```python
from build123d import *

# Parameters (mm, degrees)
BOSS_EXTRUDE1_DEPTH = 19.999999553
CUT_EXTRUDE1_DEPTH  = 158.443784597
CUT_EXTRUDE2_DEPTH  = 158.443784597
SKETCH7_W           = 15.825305434
SKETCH7_H           = 12.213007454
SKETCH7_W_2         = 10.489088449
SKETCH7_H_2         = 8.460664219
BOSS_EXTRUDE5_DEPTH = 20
SKETCH6_R           = 3.982936417
SKETCH6_R_2         = 3.990480896
CUT_EXTRUDE8_DEPTH  = 40
SKETCH8_W           = 26.734403149
SKETCH8_H           = 11.210794898
CUT_EXTRUDE9_DEPTH  = 30
FILLET1_R           = 5
FILLET2_R           = 5
SKETCH9_W           = 67.375066669
SKETCH9_H           = 11.734562751
CUT_EXTRUDE10_DEPTH = 8


with BuildPart() as part:
    # Sketch1 → Boss-Extrude1 (new body)
    with BuildSketch(Plane(origin=(0, 0, 0), x_dir=(-1, 0, 0), z_dir=(0, 0, -1))):
        Polygon((150.224894285, 11.525735259), (149.094194174, 12.437307276), (147.882685065, 13.238362968), (146.601140499, 13.921783306), (145.260930061, 14.481496066), (143.87395978, 14.912526123), (-3.873967333, 14.912526123), (-5.275767762, 14.476095326), (-6.629663985, 13.908221386), (-7.923361845, 13.214060105), (-9.145116434, 12.399914674), (-10.28383337, 11.473178864), (-11.329172179, 10.442265309), (-12.271642685, 9.316536598), (-13.102686033, 8.106213063), (-13.814756647, 6.822284777), (-14.401388355, 5.476410501), (-14.857255854, 4.080810118), (-15.178218484, 2.648155671), (-15.361363068, 1.191455987), (-15.405026264, -0.276062055), (-15.308812261, -1.741073444), (-15.073592775, -3.19027598), (-14.70150426, -4.610510543), (-14.195927419, -5.988881458), (-13.561449945, -7.312873378), (-12.803834863, -8.570464328), (-11.929960921, -9.750235826), (-10.947762057, -10.841473937), (129.052236676, -10.841473937), (130.121722817, -11.824152432), (131.278976798, -12.701761909), (132.513716817, -13.466504402), (133.815005422, -14.111584984), (135.171234608, -14.631270431), (136.570379138, -15.020942315), (137.999981642, -15.277140774), (139.447391033, -15.39758686), (140.899673104, -15.381210484), (142.343983054, -15.228157863), (143.767461181, -14.939788729), (145.157456398, -14.518666081), (146.501630545, -13.968531042), (147.788017988, -13.294272125), (149.00521934, -12.501881458), (150.142401457, -11.59839984), (151.189431548, -10.591856204), (152.137070894, -9.49119404), (152.976840734, -8.306192234), (153.701290488, -7.047383115), (154.303997755, -5.725951865), (154.779613018, -4.353639204), (155.123889446, -2.9426408), (155.333772302, -1.505494351), (155.407398939, -0.054970031), (155.344113708, 1.39604276), (155.144497752, 2.834650222), (154.81030941, 4.248069134), (154.344499111, 5.623740144), (153.751239181, 6.949439179), (153.035759926, 8.21338594), (152.204483747, 9.40434821), (151.264742017, 10.511744767), align=None)
    extrude(amount=-BOSS_EXTRUDE1_DEPTH)

    # Sketch2 → Cut-Extrude1 (cut, through all)
    with BuildSketch(Plane.XY.offset(19.999999553)):
        Polygon((3.729888937, 1.444966649), (3.400868736, 2.105728723), (2.956035547, 2.694782568), (2.410538495, 3.192068776), (1.78295339, 3.580653109), (1.094651991, 3.847302636), (0.369073445, 3.982936498), (-0.369073445, 3.982936498), (-1.094651991, 3.847302636), (-1.78295339, 3.580653109), (-2.410538495, 3.192068776), (-2.956035547, 2.694782568), (-3.400868736, 2.105728723), (-3.729888937, 1.444966649), (-3.93189257, 0.73499803), (-4.00000019, 0), (-3.93189257, -0.73499803), (-3.729888937, -1.444966649), (-3.400868736, -2.105728723), (-2.956035547, -2.694782568), (-2.410538495, -3.192068776), (-1.78295339, -3.580653109), (-1.094651991, -3.847302636), (-0.369073445, -3.982936498), (0.369073445, -3.982936498), (1.094651991, -3.847302636), (1.78295339, -3.580653109), (2.410538495, -3.192068776), (2.956035547, -2.694782568), (3.400868736, -2.105728723), (3.729888937, -1.444966649), (3.93189257, -0.73499803), (4.00000019, 0), (3.93189257, 0.73499803), align=None)
    extrude(amount=-CUT_EXTRUDE1_DEPTH, mode=Mode.SUBTRACT)

    # Sketch3 → Cut-Extrude2 (cut, through all)
    with BuildSketch(Plane.XY.offset(19.999999553)):
        Polygon((-139.630913734, 3.982936498), (-140.369072556, 3.982936498), (-141.094654799, 3.847302636), (-141.782954335, 3.580653109), (-142.41053164, 3.192068776), (-142.956033349, 2.694782568), (-143.400862813, 2.105728723), (-143.729895353, 1.444966649), (-143.931895494, 0.73499803), (-143.999993801, 0), (-143.931895494, -0.73499803), (-143.729895353, -1.444966649), (-143.400862813, -2.105728723), (-142.956033349, -2.694782568), (-142.41053164, -3.192068776), (-141.782954335, -3.580653109), (-141.094654799, -3.847302636), (-140.369072556, -3.982936498), (-139.630913734, -3.982936498), (-138.905346394, -3.847302636), (-138.217046857, -3.580653109), (-137.589469552, -3.192068776), (-137.043967843, -2.694782568), (-136.599138379, -2.105728723), (-136.270105839, -1.444966649), (-136.068105698, -0.73499803), (-136.000007391, 0), (-136.068105698, 0.73499803), (-136.270105839, 1.444966649), (-136.599138379, 2.105728723), (-137.043967843, 2.694782568), (-137.589469552, 3.192068776), (-138.217046857, 3.580653109), (-138.905346394, 3.847302636), align=None)
    extrude(amount=-CUT_EXTRUDE2_DEPTH, mode=Mode.SUBTRACT)

    # Sketch7 → Boss-Extrude5 (add)
    with BuildSketch(Plane.XY.offset(19.999999553)):
        with Locations((-139.666933083, -0.328537463)):
            Rectangle(SKETCH7_W, SKETCH7_H)
        with Locations((0.16180396, 0.00184402)):
            Rectangle(SKETCH7_W_2, SKETCH7_H_2)
    extrude(amount=-BOSS_EXTRUDE5_DEPTH)

    # Sketch6 → Cut-Extrude8 (cut)
    with BuildSketch(Plane(origin=(0, 0, -10), x_dir=(-1, 0, 0), z_dir=(0, 0, -1))):
        with Locations((4.82e-07, 8.1e-08)):
            Circle(SKETCH6_R)
        with Locations((140.006757016, -0.008937853)):
            Circle(SKETCH6_R_2)
    extrude(amount=-CUT_EXTRUDE8_DEPTH, mode=Mode.SUBTRACT)

    # Sketch8 → Cut-Extrude9 (cut)
    with BuildSketch(Plane.XY.offset(19.999999553)):
        with Locations((-96.813347326, 9.307128674)):
            Rectangle(SKETCH8_W, SKETCH8_H)
    extrude(amount=-CUT_EXTRUDE9_DEPTH, mode=Mode.SUBTRACT)

    # Fillet1
    fillet1_edges = [part.edges().sort_by_distance(p)[0] for p in [
        (-83.446145751, 3.701731225, 9.999999776),
        (-110.1805489, 3.701731225, 9.999999776),
    ]]
    fillet(fillet1_edges, radius=FILLET1_R)

    # Fillet2
    fillet2_edges = [part.edges().sort_by_distance(p)[0] for p in [
        (-83.446145751, 14.912526123, 9.999999776),
        (-110.1805489, 14.912526123, 9.999999776),
    ]]
    fillet(fillet2_edges, radius=FILLET2_R)

    # Sketch9 → Cut-Extrude10 (cut)
    with BuildSketch(Plane(origin=(0, 2.549240283, 0), x_dir=(-1, 0, 0), z_dir=(0, 0, -1))):
        with Locations((40.062197326, -0.800943257)):
            Rectangle(SKETCH9_W, SKETCH9_H)
    extrude(amount=-CUT_EXTRUDE10_DEPTH, mode=Mode.SUBTRACT)


solid = part.part
```
Could you check a few things on this model? Use its own coordinates, in mm. A direction names the side the tool comes from. Round coordinates to 2 decimals unless told otherwise and drop trailing zeros. Order: outer loops, then holes, each group sorted by start corner. A loop starts at its lowest first (then second) coordinate and runs counter-clockwise, first axis right, second up. Notation, with made-up numbers: M -25.75,-14.75 L 2.25,-14.75 A23 cw 2.25,-6.75 Z; hole C 34,18.5 d1. An arc over 180 degrees is marked long. One line per question, with ' | ' between items. Start each with the question number.
(1) Suppose I cut it at C-C on z = 16. Count the separate pieces of the cut face and the enclosed holes in it, then the cut area to 3 significant figures.
(2) Suppose I cut it at A-A on x = 0. List the corners of the cut face in (y, z) for me.
(3) For faces 1 (the face through (-136.02, 0.17, 9.86)), 2 (the face through (-40, 2, 8)), 3 (the face through (-58, -10.841, 10)), 4 (the face through (-97, 3.702, 10)), which set-ups out of +Z, -Z, +X, -X, +Y, -Y let a thin tool reach every point of the face, with its end or its side?
(4) Thinking about a two-plate mould opening in Y: for faces 5 (the face through (-69, 0, 20)), 6 (the face through (0.86, -3.89, 9.86)), 7 (the face through (-130, 14.913, 10)), which applies, +Y half, -Y half, draft (parallel to the pull), parting line (faces both ways), or undercut?
(5) For P1, Ø9, axis at x = -56.5, z = 5, coming from the -Y side; P2, Ø4, axis at y = -10, z = 16, coming from the -X side; P3, Ø6, axis at y = 8, z = 6.5, coming from the +X side; P4, Ø7, axis at x = -140.01, y = -0.01, coming from the +Z side, each with a flat end and sliding along its axis, tell me the tip position at first contact or that it passes through.
(6) Suppose I cut it at B-B on x = -51. List the corners of the cut face in (y, z) for me, then the cut area to 3 significant figures.
(7) Please list where these lines run through material, in increasing order: line 1 along Y through (x, z) = (-19.5, 3.25); line 2 along Y through (x, z) = (0, 7.5); line 3 along X through (y, z) = (1.5, 17.5).
Geometry results:
1) separate pieces: 1 | enclosed holes: 2 | area: 3,950 mm²
2) outline: M -10.84,0 L -3.98,0 L -3.98,20 L -10.84,20 Z; M 3.98,0 L 14.91,0 L 14.91,20 L 3.98,20 Z
3) face 1: +Z, -Z | face 2: -Z | face 3: +Z, -Z, +X, -Y | face 4: +Z, -Z, +Y
4) face 5: draft | face 6: undercut | face 7: +Y half
5) P1: y = -10.84 | P2: x = -153.15 | P3: x = 14.56 | P4: through
6) outline: M -10.84,0 L -4.12,0 L -4.12,8 L 7.62,8 L 7.62,0 L 14.91,0 L 14.91,20 L -10.84,20 Z | area: 421 mm²
7) line 1: -10.84 to -4.12, 7.62 to 14.91 | line 2: -10.84 to -3.98, 3.98 to 14.91 | line 3: -155.33 to -143.7, -136.31 to -3.69, 3.69 to 15.32
